from build123d import *

# Parameters (mm, degrees)
BOSS_EXTRUDE1_DEPTH = 15
SKETCH2_R           = 5
BOSS_EXTRUDE2_DEPTH = 150


with BuildPart() as part:
    # Sketch1 → Boss-Extrude1 (new body)
    with BuildSketch(Plane.XY):
        with BuildLine():
            Line((-9, 0), (-9, 65))
            ThreePointArc((-9, 65), (0, 74), (9, 65))
            Line((9, 65), (9, 0))
            ThreePointArc((9, 0), (0, -9), (-9, 0))
        make_face()
        with BuildLine():
            Line((-4, 0), (-4, 65))
            ThreePointArc((-4, 65), (0, 69), (4, 65))
            Line((4, 65), (4, 0))
            ThreePointArc((4, 0), (0, -4), (-4, 0))
        make_face(mode=Mode.SUBTRACT)
    extrude(amount=BOSS_EXTRUDE1_DEPTH)

    # Sketch2 → Boss-Extrude2 (add)
    with BuildSketch(Plane(origin=(9, 0, 0), x_dir=(0, 0, -1), z_dir=(1, 0, 0))):
        with Locations(Location((-7.5, 32.5, 0), (0, 0, 180))):
            Circle(SKETCH2_R)
    boss_extrude2 = extrude(amount=BOSS_EXTRUDE2_DEPTH)

    # Mirror1: Boss-Extrude2 across plane
    add(boss_extrude2.mirror(Plane(origin=(0, 0, 0), x_dir=(0, 0, 1), z_dir=(1, 0, 0))))


solid = part.part
The listing builds one solid part. Answer for the finished solid, in the listing's coordinates (mm). A direction names the side the tool comes from. Give positions to 0.01 mm unless a question says otherwise; leave off trailing zeros. Write each loop counter-clockwise with the first axis right and the second up, starting at its lowest first coordinate (ties: lowest second). Pieces come first, ordered by that corner, then holes. Notation, with made-up numbers: (54.25, 75.25) -> (58.25, 75.25) arc R24 ccw to (58.25, 111.25) -> close; hole circle Ø10 at (57, 51.25). An arc over 180 degrees is marked (long way). Use a Markdown table: item, result.
(1) For faces 5 (the cylindrical face through (82.95, 37.38, 6.42)), 6 (the flat face through (159, 32, 7)), 7 (the flat face through (-4, 32, 7)), determine the directions among +Z, -Z, +X, -X, +Y, -Y from which every point of the face is accessible in a straight line to the end or side of a thin tool.
Return value:
| item | result |
|---|---|
| face 5 | +X |
| face 6 | +Z, -Z, +X, +Y, -Y |
| face 7 | +Z, -Z |
(2) Flat-ended cylindrical pins translate along their axes: P1, Ø8, axis at x = -9, y = 12, coming from the -Z side; P2, Ø1, axis at x = -59, z = 3, coming from the -Y side; P3, Ø5, axis at y = 50, z = 7.5, coming from the -X side; P4, Ø3, axis at x = 87, z = 3, coming from the +Y side. Find the tip coordinate at first contact, or state that the pin passes through.
Return value:
| item | result |
|---|---|
| P1 | z = 0 |
| P2 | y = 29.5 |
| P3 | x = -9 |
| P4 | y = 36.5 |
(3) Section B-B, the plane x = 0 is taken. Determine the outline of the cut face in (y, z).
Return value:
| item | result |
|---|---|
| outline | (-9, 0) -> (-4, 0) -> (-4, 15) -> (-9, 15) -> close; (69, 0) -> (74, 0) -> (74, 15) -> (69, 15) -> close |
(4) Determine the mould class of faces 1 (the cylindrical face through (-82.95, 37.38, 6.42)), 2 (the cylindrical face through (0, -4, 7)), 3 (the flat face through (-159, 32, 7)), 4 (the cylindrical face through (0, -9, 7)) for opening direction Y: released by +Y, released by -Y, zero draft, split by the parting line, or undercut.
Return value:
| item | result |
|---|---|
| face 1 | split by the parting line |
| face 2 | undercut |
| face 3 | zero draft |
| face 4 | released by -Y |
(5) Section D-D, the plane y = 44.5 is taken. Determine the outline of the cut face in (x, z).
Return value:
| item | result |
|---|---|
| outline | (-9, 0) -> (-4, 0) -> (-4, 15) -> (-9, 15) -> close; (4, 0) -> (9, 0) -> (9, 15) -> (4, 15) -> close |
(6) Section C-C, the plane z = 7.5 is taken. Determine the outline of the cut face in (x, y), then the cut area to 3 significant figures.
Return value:
| item | result |
|---|---|
| outline | (-159, 27.5) -> (-9, 27.5) -> (-9, 0) arc R9 ccw to (9, 0) -> (9, 27.5) -> (159, 27.5) -> (159, 37.5) -> (9, 37.5) -> (9, 65) arc R9 ccw to (-9, 65) -> (-9, 37.5) -> (-159, 37.5) -> close; hole (-4, 0) arc R4 ccw to (4, 0) -> (4, 65) arc R4 ccw to (-4, 65) -> close |
| area | 3,850 mm2 |
(7) Section A-A, the plane y = 32.5 is taken. Determine the outline of the cut face in (x, z).
Return value:
| item | result |
|---|---|
| outline | (-159, 2.5) -> (-9, 2.5) -> (-9, 0) -> (-4, 0) -> (-4, 15) -> (-9, 15) -> (-9, 12.5) -> (-159, 12.5) -> close; (4, 0) -> (9, 0) -> (9, 2.5) -> (159, 2.5) -> (159, 12.5) -> (9, 12.5) -> (9, 15) -> (4, 15) -> close |
(8) Find the intervals of material crossed by probe 1 along X at (y, z) = (40, 5.25); probe 2 along X at (y, z) = (35, 6.25); probe 3 along Y at (x, z) = (52.5, 3.75), in increasing order. Write a range as from..to.
Return value:
| item | result |
|---|---|
| probe 1 | -9..-4, 4..9 |
| probe 2 | -159..-4, 4..159 |
| probe 3 | 29.19..35.81 |
